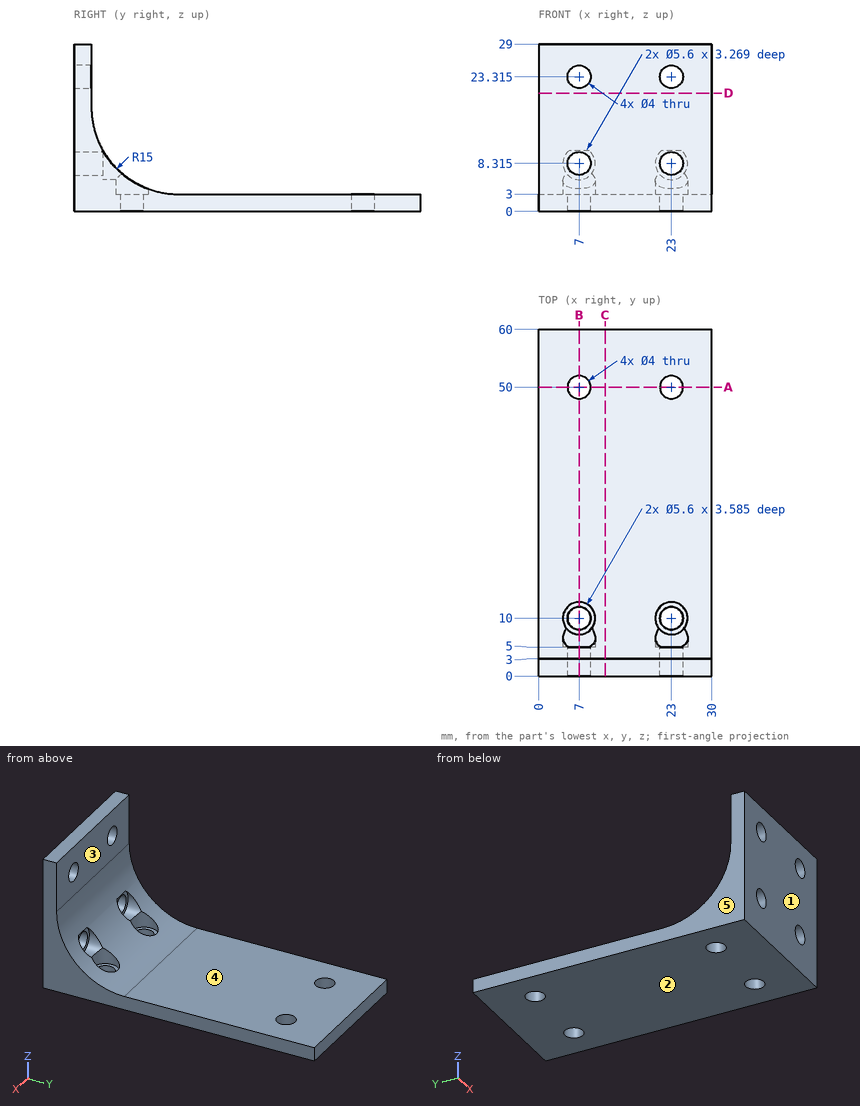
Here's the drawing with two shaded views (mm, measured from the low corner). I have some questions. A direction names the side the tool comes from. Give positions to 0.01 mm unless a question says otherwise; leave off trailing zeros. Loops run counter-clockwise (first coordinate to the right, second up) from the corner with the lowest first, then second, coordinate; pieces in that order, holes last. Notation, with made-up numbers: M 62,61.5 L 68,61.5 A11 ccw 68,69.5 Z; hole C 82.5,-8 d11. An arc over 180 degrees is marked long. Use one line per item in the form item = value. Start each with the question number.
Q1. Will these pins go through, and if not, where does the flat tip stop? pin 1 Ø3.5 at (x, z) = (23, 8.32) entering from -Y; pin 2 Ø5 at (x, y) = (13, 39.5) entering from -Z; pin 3 Ø9 at (x, y) = (7, 10) entering from +Z; pin 4 Ø4.5 at (x, y) = (23, 50) entering from +Z.
Q2. Which directions (+Z, -Z, +X, -X, +Y, -Y) give clear straight access to the entire face, cutting with the end or side of a thin tool? Please do the marked faces 4 and 5.
Q3. If we section it at A-A (y = 50): Write out the boundary of the cut face in (x, z).
Q4. I need wall thicknesses on line 1 along Y through (x, z) = (7, 1.85); line 2 along X through (y, z) = (10, 4.4); line 3 along Y through (x, z) = (4, 25.5). Which ranges of each line are inside material? Lowest first, please.
Q5. If we section it at B-B (x = 7): State how many separate pieces and enclosed holes the cut face has, then the cut area to 3 significant figures.
Q6. If we section it at C-C (x = 11.5): Write out the boundary of the cut face in (y, z), then the cut area to 3 significant figures.
Q7. Thinking about a two-plate mould opening in Y: for the marked faces 1, 2 and 3, which applies, +Y half, -Y half, draft (parallel to the pull), parting line (faces both ways), or undercut?
Q8. If we section it at D-D (z = 20.5): Write out the boundary of the cut face in (x, y).
Taken from the geometry:
q1.pin_1 = through
q1.pin_2 = 0
q1.pin_3 = 8.4
q1.pin_4 = 3
q2.face_4 = +Z, +X, -X, +Y
q2.face_5 = +Z, -Z, -X, +Y, -Y
q3.outline = M 0,0 L 5,0 L 5,3 L 0,3 Z; M 9,0 L 21,0 L 21,3 L 9,3 Z; M 25,0 L 30,0 L 30,3 L 25,3 Z
q4.line_1 = 0 to 8, 12 to 48, 52 to 60
q4.line_2 = 0 to 4.2, 9.8 to 20.2, 25.8 to 30
q4.line_3 = 0 to 3
q5.separate_pieces = 5
q5.enclosed_holes = 0
q5.area = 229 mm^2
q6.outline = M 0,0 L 60,0 L 60,3 L 18,3 A15 cw 3,18 L 3,29 L 0,29 Z
q6.area = 306 mm^2
q7.face_1 = -Y half
q7.face_2 = draft
q7.face_3 = +Y half
q8.outline = M 0,0 L 30,0 L 30,3 L 0,3 Z
